Build history of the part. All positions in model axes, mm. Face numbers are marked on the shaded views. Round coordinates to 2 decimals unless told otherwise and drop trailing zeros. Write each loop counter-clockwise with the first axis right and the second up, starting at its lowest first coordinate (ties: lowest second). Pieces come first, ordered by that corner, then holes. Notation, with made-up numbers: (46, -32.5) - (98, -32.5) arc R11 ccw to (98, -20.5) - close; hole circle Ø4 at (30.25, 21). An arc over 180 degrees is marked (long way). One line per question, with ' | ' between items.
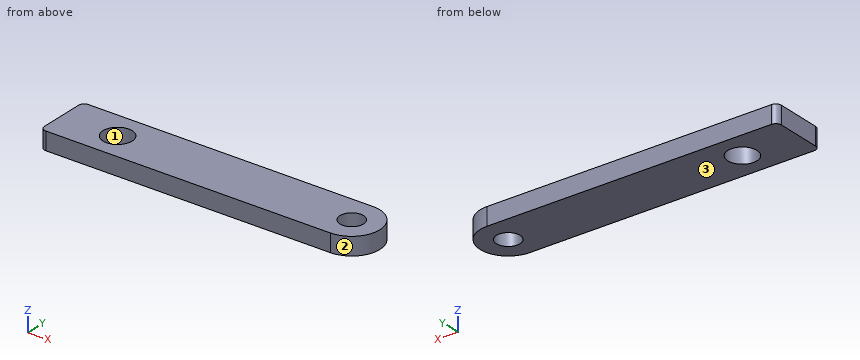
from build123d import *

# Parameters (mm, degrees)
BOSS_EXTRUDE1_DEPTH        = 3.175
F_4_2_4_2_DIAMETER_HOLE1_D = 4.2
F_5_2_5_2_DIAMETER_HOLE1_D = 5.2


with BuildPart() as part:
    # Sketch1 → Boss-Extrude1 (new body)
    with BuildSketch(Plane.XY.offset(3.175)):
        with BuildLine():
            Line((0, 9), (0, 1))
            ThreePointArc((0, 1), (0.292893219, 0.292893219), (1, 0))
            Line((1, 0), (51.75, 0))
            ThreePointArc((51.75, 0), (56.75, 5), (51.75, 10))
            Line((51.75, 10), (1, 10))
            ThreePointArc((1, 10), (0.292893219, 9.707106781), (0, 9))
        make_face()
    extrude(amount=-BOSS_EXTRUDE1_DEPTH)

    # Ø4.2 (4.2) Diameter Hole1 (through all)
    with Locations(Plane.XY.offset(3.175)):
        with Locations((51.75, 5)):
            Hole(F_4_2_4_2_DIAMETER_HOLE1_D / 2)

    # Ø5.2 (5.2) Diameter Hole1 (through all)
    with Locations(Plane.XY.offset(3.175)):
        with Locations((10, 5)):
            Hole(F_5_2_5_2_DIAMETER_HOLE1_D / 2)


solid = part.part
Q1. Pull direction X, two halves, no side cores. Call the marked faces 1, 2 and 3: +X half, -X half, draft (parallel to the pull), parting line (faces both ways), or undercut.
Found:
face 1: undercut | face 2: +X half | face 3: draft
Q2. Drill centre lines: L1, parallel to Y at x = 51.75, z = 0.75; L2, parallel to Y at x = 10, z = 2.45; L3, parallel to X at y = 3.75, z = 2.25. Where is each one in solid material? Low to high. Write a range as from..to.
Found:
L1: 0..2.9, 7.1..10 | L2: 0..2.4, 7.6..10 | L3: 0..7.72, 12.28..50.06, 53.44..56.59
Q3. Saw through at C-C, the plane z = 2.7. List the corners of the cut face in (x, y).
Found:
outline: (0, 1) arc R1 ccw to (1, 0) - (51.75, 0) arc R5 ccw to (51.75, 10) - (1, 10) arc R1 ccw to (0, 9) - close; hole circle Ø5.2 at (10, 5); hole circle Ø4.2 at (51.75, 5)
Q4. Saw through at A-A, the plane x = 10. List the corners of the cut face in (y, z) (3 decimals).
Found:
outline: (0, 0) - (2.4, 0) - (2.4, 3.175) - (0, 3.175) - close; (7.6, 0) - (10, 0) - (10, 3.175) - (7.6, 3.175) - close
Q5. Saw through at B-B, the plane y = 5. List the corners of the cut face in (x, z) (3 decimals).
Found:
outline: (0, 0) - (7.4, 0) - (7.4, 3.175) - (0, 3.175) - close; (12.6, 0) - (49.65, 0) - (49.65, 3.175) - (12.6, 3.175) - close; (53.85, 0) - (56.75, 0) - (56.75, 3.175) - (53.85, 3.175) - close
